```python
from build123d import *

# Parameters (mm, degrees)
SKETCH1_W           = 43
SKETCH1_H           = 60
SKETCH1_R           = 1.5875
BOSS_EXTRUDE1_DEPTH = 2.54
SKETCH2_W           = 50.5
SKETCH2_H           = 46
BOSS_EXTRUDE2_DEPTH = 17.65


with BuildPart() as part:
    # Sketch1 → Boss-Extrude1 (new body)
    with BuildSketch(Plane(origin=(0, 0, 0), x_dir=(1, 0, 0), z_dir=(0, 1, 0))):
        Rectangle(SKETCH1_W, SKETCH1_H)
        with Locations(Location((-18.4, 26.5, 0), (0, 0, 270))):
            Circle(SKETCH1_R, mode=Mode.SUBTRACT)
        with Locations(Location((18.4, 26.5, 0), (0, 0, 270))):
            Circle(SKETCH1_R, mode=Mode.SUBTRACT)
        with Locations(Location((18.4, -26.5, 0), (0, 0, 270))):
            Circle(SKETCH1_R, mode=Mode.SUBTRACT)
        with Locations(Location((-18.4, -26.5, 0), (0, 0, 270))):
            Circle(SKETCH1_R, mode=Mode.SUBTRACT)
    extrude(amount=BOSS_EXTRUDE1_DEPTH)

    # Sketch2 → Boss-Extrude2 (add)
    with BuildSketch(Plane(origin=(0, 2.54, 0), x_dir=(1, 0, 0), z_dir=(0, 1, 0))):
        Rectangle(SKETCH2_W, SKETCH2_H)
    extrude(amount=BOSS_EXTRUDE2_DEPTH)


solid = part.part
```
CAD build for the part. Positions are in the model's coordinates, mm. A direction names the side the tool comes from. Coordinates: 2 decimals unless noted, no trailing zeros. Write each loop counter-clockwise with the first axis right and the second up, starting at its lowest first coordinate (ties: lowest second). Pieces come first, ordered by that corner, then holes.
(1) Cut at D-D, the plane z = -10.5. List the corners of the cut face in (x, y), and give its area (3 significant figures).
(2) Drill centre lines: probe 1 along X at (y, z) = (1, 26.5); probe 2 along Z at (x, y) = (1, 17.75); probe 3 along Y at (x, z) = (23, 4). Where is each one in solid material? Low to high.
(3) Two-plate mould, pull along Z, no slides. Class faces 1 (the face through (19.74, 1.25, -25.65)), 2 (the face through (0, 1, 30)), 3 (the face through (0, 2.54, -27)): +Z half, -Z half, draft (parallel to the pull), parting line (faces both ways), or undercut.
(4) 3-axis set-ups, long thin cutter, end or side, ignore diameter. For faces 4 (the face through (-23, 2.54, 0)), 5 (the face through (21.5, 1, 0)), 6 (the face through (-25.25, 11, 0)), 7 (the face through (0, 11, -23)), 8 (the face through (0, 11, 23)): which of +Z, -Z, +X, -X, +Y, -Y reach the whole face in a straight line?
(5) Cut at B-B, the plane x = -18.4. List the corners of the cut face in (y, z).
(6) Flat gauge pins, fed straight in: pin 1 (8 mm diameter, centred on x = -10, y = 12.5, fed in from +Z); pin 2 (1.9 mm diameter, centred on x = -23, z = 6.5, fed in from -Y); pin 3 (5 mm diameter, centred on x = -18.4, z = 26.5, fed in from +Y). Where does each tip first touch, or does it go through?
(7) Cut at C-C, the plane y = 1.5. List the corners of the cut face in (x, z) (1 decimal).
(8) Cut at A-A, the plane z = 26.5. List the corners of the cut face in (x, y).
Geometry says:
1. outline: (-25.25, 2.54) - (-21.5, 2.54) - (-21.5, 0) - (21.5, 0) - (21.5, 2.54) - (25.25, 2.54) - (25.25, 20.19) - (-25.25, 20.19) - close
1. area: 1,000 mm2
2. probe 1: x = -21.5 to -19.99, -16.81 to 16.81, 19.99 to 21.5
2. probe 2: z = -23 to 23
2. probe 3: y = 2.54 to 20.19
3. face 1: undercut
3. face 2: +Z half
3. face 3: draft
4. face 4: +Z, -Z, -X, -Y
4. face 5: +Z, -Z, +X, -Y
4. face 6: +Z, -Z, -X, +Y, -Y
4. face 7: -Z, +X, -X, +Y
4. face 8: +Z, +X, -X, +Y
5. outline: (0, -30) - (2.54, -30) - (2.54, -28.09) - (0, -28.09) - close; (0, -24.91) - (2.54, -24.91) - (2.54, -23) - (20.19, -23) - (20.19, 23) - (2.54, 23) - (2.54, 24.91) - (0, 24.91) - close; (0, 28.09) - (2.54, 28.09) - (2.54, 30) - (0, 30) - close
6. pin 1: stops at z = 23
6. pin 2: stops at y = 2.54
6. pin 3: stops at y = 2.54
7. outline: (-21.5, -30) - (21.5, -30) - (21.5, 30) - (-21.5, 30) - close; hole circle Ø3.2 at (-18.4, -26.5); hole circle Ø3.2 at (-18.4, 26.5); hole circle Ø3.2 at (18.4, -26.5); hole circle Ø3.2 at (18.4, 26.5)
8. outline: (-21.5, 0) - (-19.99, 0) - (-19.99, 2.54) - (-21.5, 2.54) - close; (-16.81, 0) - (16.81, 0) - (16.81, 2.54) - (-16.81, 2.54) - close; (19.99, 0) - (21.5, 0) - (21.5, 2.54) - (19.99, 2.54) - close
